The model under review builds one solid part; all positions refer to its coordinate system, in mm. A direction names the side the tool comes from. Coordinates: 2 decimals unless noted, no trailing zeros. Order: outer loops, then holes, each group sorted by start corner. A loop starts at its lowest first (then second) coordinate and runs counter-clockwise, first axis right, second up.
from build123d import *

# Parameters (mm, degrees)
SKETCH1_R           = 3.5
BOSS_EXTRUDE1_DEPTH = 4.5


with BuildPart() as part:
    # Sketch1 → Boss-Extrude1 (new body)
    with BuildSketch(Plane(origin=(0, 0, 0), x_dir=(1, 0, 0), z_dir=(0, 1, 0))):
        with BuildLine():
            Line((11, 7), (30, 7))
            ThreePointArc((30, 7), (37, 0), (30, -7))
            Line((30, -7), (0, -7))
            ThreePointArc((0, -7), (-4.949747468, -4.949747468), (-7, 0))
            Line((-7, 0), (-7, 21.7))
            Line((-7, 21.7), (-7, 56.2))
            ThreePointArc((-7, 56.2), (-3, 60.2), (1, 56.2))
            Line((1, 56.2), (1, 17))
            ThreePointArc((1, 17), (3.928932188, 9.928932188), (11, 7))
        make_face()
        with Locations(Location((0, 0, 0), (0, 0, 270))):
            Circle(SKETCH1_R, mode=Mode.SUBTRACT)
        with Locations(Location((30, 0, 0), (0, 0, 270))):
            Circle(SKETCH1_R, mode=Mode.SUBTRACT)
        with BuildLine():
            Line((-5, 21.7), (-5, 23.7))
            ThreePointArc((-5, 23.7), (-3, 25.7), (-1, 23.7))
            Line((-1, 23.7), (-1, 21.7))
            ThreePointArc((-1, 21.7), (-3, 19.7), (-5, 21.7))
        make_face(mode=Mode.SUBTRACT)
        with BuildLine():
            Line((-5, 36.2), (-5, 38.2))
            ThreePointArc((-5, 38.2), (-3, 40.2), (-1, 38.2))
            Line((-1, 38.2), (-1, 36.2))
            ThreePointArc((-1, 36.2), (-3, 34.2), (-5, 36.2))
        make_face(mode=Mode.SUBTRACT)
        with BuildLine():
            Line((-5, 54.2), (-5, 56.2))
            ThreePointArc((-5, 56.2), (-3, 58.2), (-1, 56.2))
            Line((-1, 56.2), (-1, 54.2))
            ThreePointArc((-1, 54.2), (-3, 52.2), (-5, 54.2))
        make_face(mode=Mode.SUBTRACT)
    extrude(amount=BOSS_EXTRUDE1_DEPTH)


solid = part.part
(1) Tool access review of faces 4 (the face through (-3, 2.2, -19.7)), 5 (the face through (2, 4.5, -12)): name each direction out of +Z, -Z, +X, -X, +Y, -Y from which nothing blocks a thin tool from reaching the whole face with its end or side.
(2) Consider section B-B (z = -2.5). Give the boundary of the cut face in (x, y), then the cut area to 3 significant figures.
(3) Wall thickness on line 1 (Z direction, x = -1.5, y = 3.75); line 2 (X direction, y = 1.95, z = -30.5); line 3 (Z direction, x = 21.5, y = 2.95): over which ranges is each line inside the solid? List them lowest first.
(4) Insertion check: pin 1 Ø2 at (y, z) = (0.5, -31) entering from +X; pin 2 Ø1.3 at (x, y) = (23, 3) entering from -Z. Each pin has a flat end and moves straight along its axis. Give the tip position at first contact, or say it passes through.
(5) Consider section A-A (y = 1.05). Give the boundary of the cut face in (x, z).
(6) Consider section D-D (z = -14). Give the boundary of the cut face in (x, y), then the cut area to 3 significant figures.
(7) The part is to be moulded in two halves that separate along X. For faces 1 (the face through (-3.417, 2.218, -0.759)), 2 (the face through (20, 2, -7)), 3 (the face through (37, 2, 0)), say which applies: +X half, -X half, draft (parallel to the pull), parting line (faces both ways), or undercut.
(8) Consider section C-C (x = 29). Give the boundary of the cut face in (y, z), then the cut area to 3 significant figures.
Findings:
1. face 4: +Y, -Y
1. face 5: +Z, -Z, +X, -X, +Y
2. outline: (-7, 0) - (-2.45, 0) - (-2.45, 4.5) - (-7, 4.5) - close; (2.45, 0) - (27.55, 0) - (27.55, 4.5) - (2.45, 4.5) - close; (32.45, 0) - (36.54, 0) - (36.54, 4.5) - (32.45, 4.5) - close
2. area: 152 mm2
3. line 1: z = -59.91 to -57.52, -52.88 to -39.52, -34.88 to -25.02, -20.38 to -3.16, 3.16 to 6.84
3. line 2: x = -7 to 1
3. line 3: z = -7 to 7
4. pin 1: stops at x = 1
4. pin 2: stops at z = -7
5. outline: (-7, -56.2) arc R4 ccw to (1, -56.2) - (1, -17) arc R10 cw to (11, -7) - (30, -7) arc R7 ccw to (30, 7) - (0, 7) arc R7 ccw to (-7, 0) - close; hole (-5, -56.2) arc R2 ccw to (-1, -56.2) - (-1, -54.2) arc R2 ccw to (-5, -54.2) - close; hole (-5, -38.2) arc R2 ccw to (-1, -38.2) - (-1, -36.2) arc R2 ccw to (-5, -36.2) - close; hole (-5, -23.7) arc R2 ccw to (-1, -23.7) - (-1, -21.7) arc R2 ccw to (-5, -21.7) - close; hole circle Ø7 at (0, 0); hole circle Ø7 at (30, 0)
6. outline: (-7, 0) - (1.46, 0) - (1.46, 4.5) - (-7, 4.5) - close
6. area: 38.1 mm2
7. face 1: undercut
7. face 2: draft
7. face 3: +X half
8. outline: (0, -7) - (4.5, -7) - (4.5, -3.35) - (0, -3.35) - close; (0, 3.35) - (4.5, 3.35) - (4.5, 7) - (0, 7) - close
8. area: 32.8 mm2
